```python
from build123d import *

# Parameters (mm, degrees)
BOSS_EXTRUDE1_DEPTH      = 3.8
CHAMFER1_SIZE            = 0.5
CHAMFER1_SIZE2           = 16.846754467
BOSS_EXTRUDE2_DEPTH      = 0.1
BOSS_EXTRUDE2_DEPTH_BACK = 3.9
SKETCH3_R                = 0.15
SKETCH4_W                = 7
SKETCH4_H                = 1
CUT_EXTRUDE2_DEPTH       = 10
FILLET1_R                = 0.1
FILLET2_R                = 0.3
FILLET3_R                = 0.2


with BuildPart() as part:
    # Sketch1 → Boss-Extrude1 (new body)
    with BuildSketch(Plane.XY):
        Polygon((0, 0), (0, 1.230198096), (17.386664873, 5.888940908), (17.464310587, 5.59916316), (0.3, 1), (0.3, 0), align=None)
    extrude(amount=BOSS_EXTRUDE1_DEPTH)

    # Chamfer1
    chamfer1_edges = [part.edges().sort_by_distance(p)[0] for p in [
        (17.42548773, 5.744052034, 3.8),
        (17.42548773, 5.744052034, 0),
    ]]
    chamfer1_side = [part.faces().sort_by_distance(p)[0] for p in [
        (17.42548773, 5.744052034, 1.9),
    ]]
    chamfer(chamfer1_edges, length=CHAMFER1_SIZE, length2=CHAMFER1_SIZE2, reference=chamfer1_side[0])

    # Sketch3 → Boss-Extrude2 (add, two sides: drawn at the far end of the back side and taken through both)
    with BuildSketch(Plane.XY.offset(3.8).offset(-BOSS_EXTRUDE2_DEPTH_BACK)):
        with Locations((0.15, 0.5)):
            Circle(SKETCH3_R)
    extrude(amount=BOSS_EXTRUDE2_DEPTH + BOSS_EXTRUDE2_DEPTH_BACK)

    # Sketch4 → Cut-Extrude2 (cut)
    with BuildSketch(Plane.XZ):
        with Locations((3.5, 1.9)):
            Rectangle(SKETCH4_W, SKETCH4_H)
    extrude(amount=-CUT_EXTRUDE2_DEPTH, mode=Mode.SUBTRACT)

    # Fillet1
    fillet1_edges = [part.edges().sort_by_distance(p)[0] for p in [
        (0, 1.230198096, 3.1),
        (0.3, 1, 3.1),
        (0, 1.230198096, 0.7),
        (0.3, 1, 0.7),
    ]]
    fillet(fillet1_edges, radius=FILLET1_R)

    # Fillet2
    fillet2_edges = [part.edges().sort_by_distance(p)[0] for p in [
        (17.42548773, 5.744052034, 0.5),
        (17.42548773, 5.744052034, 3.3),
    ]]
    fillet(fillet2_edges, radius=FILLET2_R)

    # Fillet3
    fillet3_edges = [part.edges().sort_by_distance(p)[0] for p in [
        (7, 2.950551016, 2.4),
        (7, 2.950551016, 1.4),
    ]]
    fillet(fillet3_edges, radius=FILLET3_R)


solid = part.part
```
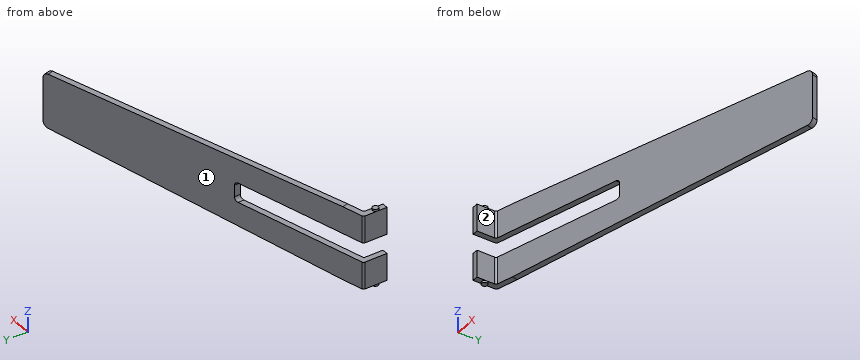
Here's how the part is built. I have some questions about the finished solid (model axes, mm). Face numbers are marked on the shaded views. A direction names the side the tool comes from. Coordinates: 2 decimals unless noted, no trailing zeros. Order: outer loops, then holes, each group sorted by start corner. A loop starts at its lowest first (then second) coordinate and runs counter-clockwise, first axis right, second up.
1) Imagine slicing it at B-B on y = 2.2. List the corners of the cut face in (x, z) for me, and give its area (3 significant figures).
2) Imagine slicing it at C-C on z = 1.05. List the corners of the cut face in (x, y) for me.
3) Imagine slicing it at D-D on y = 4.9. List the corners of the cut face in (x, z) for me (3 decimals), and give its area (3 significant figures).
4) Which directions (+Z, -Z, +X, -X, +Y, -Y) give clear straight access to the entire face, cutting with the end or side of a thin tool? Please do the marked faces 1 and 2.
5) Imagine slicing it at A-A on x = 5.5. List the corners of the cut face in (y, z) for me, and give its area (3 significant figures).
6) Will these pins go through, and if not, where does the flat tip stop? pin 1 (0.5 mm diameter, centred on y = 0, z = 0.5, fed in from +X); pin 2 (1.5 mm diameter, centred on x = 4.5, y = 2, fed in from -Z); pin 3 (2.5 mm diameter, centred on x = 3, y = 1.5, fed in from +Z).
7) I need wall thicknesses on line 1 (Y direction, x = 14.75, z = 1.7); line 2 (Y direction, x = 8.75, z = 2.05); line 3 (Z direction, x = 7.25, y = 3). Which ranges of each line are inside material? Lowest first, please.
Response values:
1. outline: (3.62, 0.08) - (4.78, 0.11) - (4.78, 1.4) - (3.62, 1.4) - close; (3.62, 2.4) - (4.78, 2.4) - (4.78, 3.69) - (3.62, 3.72) - close
1. area: 3.03 mm2
2. outline: (0, 0) - (0.3, 0) - (0.3, 0.92) arc R0.1 cw to (0.37, 1.02) - (17.46, 5.6) - (17.39, 5.89) - (0.07, 1.25) arc R0.1 ccw to (0, 1.15) - close
3. outline: (13.696, 0.387) - (14.855, 0.42) - (14.855, 3.38) - (13.696, 3.413) - close
3. area: 3.47 mm2
4. face 1: +Z, -Z, -X, +Y
4. face 2: +Z, -Z, +X, -Y
5. outline: (2.39, 0.13) - (2.7, 0.13) - (2.7, 1.4) - (2.39, 1.4) - close; (2.39, 2.4) - (2.7, 2.4) - (2.7, 3.67) - (2.39, 3.67) - close
5. area: 0.787 mm2
6. pin 1: stops at x = 0.3
6. pin 2: stops at z = 0.08
6. pin 3: stops at z = 3.78
7. line 1: y = 4.87 to 5.18
7. line 2: y = 3.26 to 3.57
7. line 3: z = 0.19 to 3.61
